from build123d import *

# Parameters (mm, degrees)
SKETCH1_W            = 63.5
SKETCH1_H            = 20
SKETCH1_R            = 1.4
BASE_DEPTH           = 8
WIRE_GROOVES_DEPTH   = 39.833780398
F_1MM_EDGE_FILLETS_R = 1


with BuildPart() as part:
    # Sketch1 → Base (new body)
    with BuildSketch(Plane(origin=(0, 0, 0), x_dir=(1, 0, 0), z_dir=(0, 1, 0))):
        Rectangle(SKETCH1_W, SKETCH1_H)
        with Locations(Location((-25.25, 0, 0), (0, 0, 270))):
            Circle(SKETCH1_R, mode=Mode.SUBTRACT)
        with Locations(Location((25.25, 0, 0), (0, 0, 90))):
            Circle(SKETCH1_R, mode=Mode.SUBTRACT)
    extrude(amount=BASE_DEPTH)

    # Sketch2 → Wire Grooves (cut, through all)
    with BuildSketch(Plane(origin=(0, 10, -10), x_dir=(1, 0, 0), z_dir=(0, 0, -1))):
        with BuildLine():
            Line((-15.5, 10), (-9.5, 10))
            ThreePointArc((-9.5, 10), (-9.997918472, 8.797918472), (-11.2, 8.3))
            Line((-11.2, 8.3), (-13.8, 8.3))
            ThreePointArc((-13.8, 8.3), (-15.002081528, 8.797918472), (-15.5, 10))
        make_face()
        with BuildLine():
            Line((9.5, 10), (15.5, 10))
            ThreePointArc((15.5, 10), (15.002081528, 8.797918472), (13.8, 8.3))
            Line((13.8, 8.3), (11.2, 8.3))
            ThreePointArc((11.2, 8.3), (9.997918472, 8.797918472), (9.5, 10))
        make_face()
    extrude(amount=-WIRE_GROOVES_DEPTH, mode=Mode.SUBTRACT)

    # 1mm Edge Fillets
    f_1mm_edge_fillets_edges = [part.edges().sort_by_distance(p)[0] for p in [
        (-31.75, 4, -10),
        (31.75, 4, -10),
        (31.75, 4, 10),
        (-31.75, 4, 10),
    ]]
    fillet(f_1mm_edge_fillets_edges, radius=F_1MM_EDGE_FILLETS_R)


solid = part.part
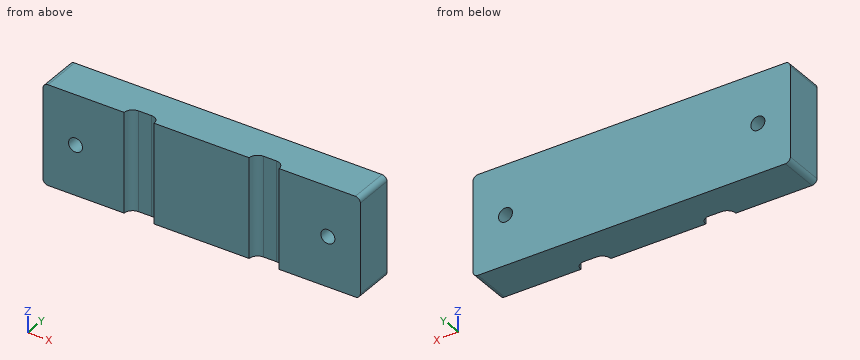
Can you work these out from the model? Positions are in its coordinate system, mm. Give positions to 0.01 mm unless a question says otherwise; leave off trailing zeros. Loops run counter-clockwise (first coordinate to the right, second up) from the corner with the lowest first, then second, coordinate; pieces in that order, holes last. Notation, with made-up numbers: (88, -25.5) -> (122, -25.5) arc R12 cw to (122, -17.5) -> close; hole circle Ø7 at (73.25, 18.25). An arc over 180 degrees is marked (long way). Write item = value, one per line.
1) Suppose I cut it at A-A on x = -25.25. Write out the boundary of the cut face in (y, z), then the cut area to 3 significant figures.
Check result:
outline = (0, -10) -> (8, -10) -> (8, -1.4) -> (0, -1.4) -> close; (0, 1.4) -> (8, 1.4) -> (8, 10) -> (0, 10) -> close
area = 138 mm2
2) Suppose I cut it at B-B on z = -2. Write out the boundary of the cut face in (x, y).
Check result:
outline = (-31.75, 0) -> (-15.5, 0) arc R1.7 cw to (-13.8, 1.7) -> (-11.2, 1.7) arc R1.7 cw to (-9.5, 0) -> (9.5, 0) arc R1.7 cw to (11.2, 1.7) -> (13.8, 1.7) arc R1.7 cw to (15.5, 0) -> (31.75, 0) -> (31.75, 8) -> (-31.75, 8) -> close
3) Will these pins go through, and if not, where does the flat tip stop? pin 1 (1.5 mm diameter, centred on x = -13.5, z = -7.5, fed in from -Y); pin 2 (0.8 mm diameter, centred on x = 12.5, z = -1.5, fed in from -Y).
Check result:
pin_1 = 1.64
pin_2 = 1.7
4) I need wall thicknesses on L1, parallel to X at y = 3.25, z = 0; L2, parallel to Z at x = 25.25, y = 3.75; L3, parallel to X at y = 0.5, z = 1.25. Which ranges of each line are inside material? Lowest first, please. Write a range as from..to.
Check result:
L1 = -31.75..-26.65, -23.85..23.85, 26.65..31.75
L2 = -10..-1.4, 1.4..10
L3 = -31.75..-25.88, -24.62..-15.42, -9.58..9.58, 15.42..24.62, 25.88..31.75
